Can you work these out from the model? Positions are in its coordinate system, mm. A direction names the side the tool comes from. Round coordinates to 2 decimals unless told otherwise and drop trailing zeros. Write each loop counter-clockwise with the first axis right and the second up, starting at its lowest first coordinate (ties: lowest second). Pieces come first, ordered by that corner, then holes. Notation, with made-up numbers: M 9.5,80.25 L 39.5,80.25 A21 ccw 39.5,92.25 Z; hole C 49.25,6 d3. An arc over 180 degrees is marked long. Answer in a Markdown table with one row per item. Add a question column.
(1) If we mould it in two halves opening along Z, with no side actions, what happens to faces 4 (the face through (-20.969, -22.972, 14.996)), 5 (the face through (-20.817, 18, 3)), 6 (the face through (20.272, -22.972, 12.306)), 7 (the face through (-26.27, 17.71, 0.57))? For each: released by +Z, released by -Z, zero draft, split by the parting line, or undercut.
(2) Suppose I cut it at C-C, the plane x = 11.5. Write out the boundary of the cut face in (y, z).
(3) If I drill on probe 1 along X at (y, z) = (9.5, 3.75); probe 2 along Y at (x, z) = (15.5, 15.5); probe 3 along X at (y, z) = (-7, 4), over which ranges is the centre line in solid material (lowest first)?
(4) Suppose I cut it at D-D, the plane y = -3.5. Write out the boundary of the cut face in (x, z), then the cut area to 4 significant figures.
(5) For faces 1 (the face through (-18.565, 17.745, 0.57)), 2 (the face through (-15.517, 17, 2)), 3 (the face through (-22.395, -23, 8)), which set-ups out of +Z, -Z, +X, -X, +Y, -Y let a thin tool reach every point of the face, with its end or its side?
(6) Suppose I cut it at B-B, the plane z = 3.75. Write out the boundary of the cut face in (x, y).
(7) I'm going to push flat-ended pins straight in: pin 1 (1.8 mm diameter, centred on x = -19.5, y = 13.5, fed in from -Z); pin 2 (5 mm diameter, centred on x = -12.21, z = 12.5, fed in from +Y); pin 3 (1.6 mm diameter, centred on x = -14, z = 3.5, fed in from +Y); pin 4 (5 mm diameter, centred on x = 15.5, y = -14, fed in from -Z). Where does each tip first touch, or does it pass through?
(8) Suppose I cut it at A-A, the plane y = 18. Count the separate pieces of the cut face and the enclosed holes in it, then the cut area to 3 significant figures.
from build123d import *

# Parameters (mm, degrees)
EXTRUDE1_DEPTH = 5
EXTRUDE2_DEPTH = 11.5
SKETCH5_R      = 1.5
EXTRUDE3_DEPTH = 4
FILLET2_R      = 5
FILLET3_R      = 4
FILLET4_R      = 5
SKETCH4_W      = 6.5
SKETCH4_H      = 4
EXTRUDE4_DEPTH = 35
FILLET1_R      = 2


with BuildPart() as part:
    # Sketch1 → Extrude1 (new body)
    with BuildSketch(Plane.XY):
        Polygon((24.583407752, -25), (24.660567061, -15), (-5.416666667, -15), (-5.416666667, 35), (-12.316666667, 35), (-12.316666667, 0), (-15.516666667, 0), (-15.516666667, 35), (-20.816666667, 35), (-20.816666667, 0), (-24.016666667, 0), (-24.016666667, 35), (-28.916666667, 35), (-28.916666667, -25), align=None)
    extrude(amount=EXTRUDE1_DEPTH)

    # Sketch3 → Extrude2 (add)
    with BuildSketch(Plane.XY.offset(5)):
        Polygon((-22.394876452, -21), (24.614271475, -21), (24.583407752, -25), (-22.394876452, -25), align=None)
    extrude(amount=EXTRUDE2_DEPTH)

    # Sketch5 → Extrude3 (cut)
    with BuildSketch(Plane(origin=(0, -21, 0), x_dir=(1, 0, 0), z_dir=(0, 1, 0))):
        with Locations(Location((-12.214752954, -12.501481725, 0), (0, 0, 270))):
            Circle(SKETCH5_R)
        with Locations(Location((18.785247046, -12.501481725, 0), (0, 0, 270))):
            Circle(SKETCH5_R)
    extrude(amount=-EXTRUDE3_DEPTH, mode=Mode.SUBTRACT)

    # Fillet2
    fillet2_edges = [part.edges().sort_by_distance(p)[0] for p in [
        (-22.394876452, -23, 16.5),
        (24.598839614, -23, 16.5),
    ]]
    fillet(fillet2_edges, radius=FILLET2_R)

    # Fillet3
    fillet3_edges = [part.edges().sort_by_distance(p)[0] for p in [
        (-5.416666667, 35, 2.5),
        (-5.416666667, -15, 2.5),
        (24.660567061, -15, 2.5),
        (-28.916666667, 35, 2.5),
    ]]
    fillet(fillet3_edges, radius=FILLET3_R)

    # Fillet4
    fillet4_edges = [part.edges().sort_by_distance(p)[0] for p in [
        (-28.916666667, -25, 2.5),
    ]]
    fillet(fillet4_edges, radius=FILLET4_R)

    # Sketch4 → Extrude4 (cut)
    with BuildSketch(Plane(origin=(0, 35, 0), x_dir=(1, 0, 0), z_dir=(0, 1, 0))):
        with Locations((-22.416666667, 0)):
            Rectangle(SKETCH4_W, SKETCH4_H)
    extrude(amount=-EXTRUDE4_DEPTH, mode=Mode.SUBTRACT)

    # Fillet1
    fillet1_edges = [part.edges().sort_by_distance(p)[0] for p in [
        (-19.166666667, 17.5, 0),
        (-25.666666667, 17.464529206, 0),
    ]]
    fillet(fillet1_edges, radius=FILLET1_R - 0.0001)  # a hair under: the kernel refuses the full size


solid = part.part
Calculated:
| question | item | result |
|---|---|---|
| 1 | face 4 | released by +Z |
| 1 | face 5 | zero draft |
| 1 | face 6 | undercut |
| 1 | face 7 | released by -Z |
| 2 | outline | M -25,0 L -15,0 L -15,5 L -21,5 L -21,16.5 L -25,16.5 Z |
| 3 | probe 1 | -28.92 to -24.02, -20.82 to -15.52, -12.32 to -5.42 |
| 3 | probe 2 | -25 to -21 |
| 3 | probe 3 | -28.92 to -5.42 |
| 4 | outline | M -28.92,0 L -5.42,0 L -5.42,5 L -28.92,5 Z |
| 4 | area | 117.5 mm² |
| 5 | face 1 | -Z, +Y |
| 5 | face 2 | +Z, -Z, +Y |
| 5 | face 3 | +Z, -X, +Y, -Y |
| 6 | outline | M -28.92,-20 A5 ccw -23.92,-25 L 24.58,-25 L 24.63,-19.03 A4 ccw 20.63,-15 L -1.42,-15 A4 cw -5.42,-11 L -5.42,31 A4 ccw -9.42,35 L -12.32,35 L -12.32,0 L -15.52,0 L -15.52,35 L -20.82,35 L -20.82,0 L -24.02,0 L -24.02,35 L -24.92,35 A4 ccw -28.92,31 Z |
| 7 | pin 1 | z = 0.61 |
| 7 | pin 2 | y = -21 |
| 7 | pin 3 | y = 0 |
| 7 | pin 4 | z = 0 |
| 8 | separate pieces | 3 |
| 8 | enclosed holes | 0 |
| 8 | area | 77.2 mm² |
